Verification items for the finished model (mm, model axes). Give positions to 0.01 mm unless a question says otherwise; leave off trailing zeros. Write each loop counter-clockwise with the first axis right and the second up, starting at its lowest first coordinate (ties: lowest second). Pieces come first, ordered by that corner, then holes. Notation, with made-up numbers: (19.5, 65.5) -> (38.5, 65.5) arc R18 cw to (38.5, 90.5) -> close; hole circle Ø11 at (-14, -17). An arc over 180 degrees is marked (long way). Write item = value, one per line.
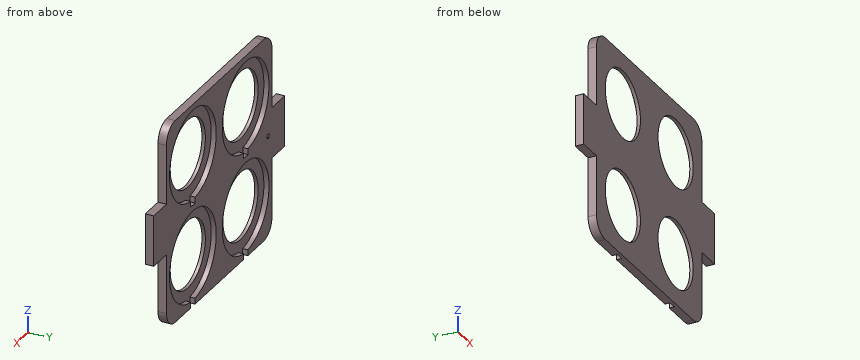
from build123d import *

# Parameters (mm, degrees)
SKETCH1_W           = 120
SKETCH1_H           = 120
BOSS_EXTRUDE1_DEPTH = 5
SKETCH2_R           = 20
CUT_EXTRUDE4_DEPTH  = 5
SKETCH3_R           = 26.6
SKETCH3_R_2         = 20
CUT_EXTRUDE5_DEPTH  = 3
SKETCH4_W           = 60
SKETCH4_H           = 5
BOSS_EXTRUDE2_DEPTH = 14.5
SKETCH5_W           = 60
SKETCH5_H           = 5
BOSS_EXTRUDE3_DEPTH = 14.5
FILLET3_R           = 10
FILLET4_R           = 10
FILLET5_R           = 10
FILLET6_R           = 10
SKETCH10_W          = 2.261137553
SKETCH10_H          = 2.574285836
CUT_EXTRUDE7_DEPTH  = 2
SKETCH12_W          = 5.377639696
SKETCH12_H          = 6.736845814
CUT_EXTRUDE10_DEPTH = 3
SKETCH14_W          = 4.90266265
SKETCH14_H          = 7.042630192
CUT_EXTRUDE11_DEPTH = 3
SKETCH15_W          = 14.5
SKETCH15_H          = 15
CUT_EXTRUDE12_DEPTH = 10


with BuildPart() as part:
    # Sketch1 → Boss-Extrude1 (new body)
    with BuildSketch(Plane(origin=(0, 0, 0), x_dir=(1, 0, 0), z_dir=(0, 1, 0))):
        Rectangle(SKETCH1_W, SKETCH1_H)
    extrude(amount=BOSS_EXTRUDE1_DEPTH)

    # Sketch2 → Cut-Extrude4 (cut)
    with BuildSketch(Plane(origin=(0, 5, 0), x_dir=(1, 0, 0), z_dir=(0, 1, 0))):
        with Locations(Location((30, 30, 0), (0, 0, 270))):
            Circle(SKETCH2_R)
        with Locations(Location((-30, -30, 0), (0, 0, 270))):
            Circle(SKETCH2_R)
        with Locations(Location((30, -30, 0), (0, 0, 270))):
            Circle(SKETCH2_R)
        with Locations(Location((-30, 30, 0), (0, 0, 270))):
            Circle(SKETCH2_R)
    extrude(amount=-CUT_EXTRUDE4_DEPTH, mode=Mode.SUBTRACT)

    # Sketch3 → Cut-Extrude5 (cut)
    # profile 1 of 4: a face of its own
    with BuildSketch(Plane(origin=(0, 5, 0), x_dir=(1, 0, 0), z_dir=(0, 1, 0))):
        with Locations(Location((30, 30, 0), (0, 0, 270))):
            Circle(SKETCH3_R)
        with Locations(Location((30, 30, 0), (0, 0, 270))):
            Circle(SKETCH3_R_2, mode=Mode.SUBTRACT)
    # profile 2 of 4: a face of its own
    with BuildSketch(Plane(origin=(0, 5, 0), x_dir=(1, 0, 0), z_dir=(0, 1, 0))):
        with Locations(Location((-30, -30, 0), (0, 0, 270))):
            Circle(SKETCH3_R)
        with Locations(Location((-30, -30, 0), (0, 0, 270))):
            Circle(SKETCH3_R_2, mode=Mode.SUBTRACT)
    # profile 3 of 4: a face of its own
    with BuildSketch(Plane(origin=(0, 5, 0), x_dir=(1, 0, 0), z_dir=(0, 1, 0))):
        with Locations(Location((30, -30, 0), (0, 0, 270))):
            Circle(SKETCH3_R)
        with Locations(Location((30, -30, 0), (0, 0, 270))):
            Circle(SKETCH3_R_2, mode=Mode.SUBTRACT)
    # profile 4 of 4: a face of its own
    with BuildSketch(Plane(origin=(0, 5, 0), x_dir=(1, 0, 0), z_dir=(0, 1, 0))):
        with Locations(Location((-30, 30, 0), (0, 0, 270))):
            Circle(SKETCH3_R)
    extrude(amount=-CUT_EXTRUDE5_DEPTH, mode=Mode.SUBTRACT)

    # Sketch4 → Boss-Extrude2 (add)
    with BuildSketch(Plane(origin=(60, 0, 0), x_dir=(0, 0, -1), z_dir=(1, 0, 0))):
        with Locations((0, 2.5)):
            Rectangle(SKETCH4_W, SKETCH4_H)
    extrude(amount=BOSS_EXTRUDE2_DEPTH)

    # Sketch5 → Boss-Extrude3 (add)
    with BuildSketch(Plane.ZY.offset(60)):
        with Locations((0, 2.5)):
            Rectangle(SKETCH5_W, SKETCH5_H)
    extrude(amount=BOSS_EXTRUDE3_DEPTH)

    # Fillet3
    fillet3_edges = [part.edges().sort_by_distance(p)[0] for p in [
        (-60, 2.5, 60),
    ]]
    fillet(fillet3_edges, radius=FILLET3_R)

    # Fillet4
    fillet4_edges = [part.edges().sort_by_distance(p)[0] for p in [
        (60, 2.5, 60),
    ]]
    fillet(fillet4_edges, radius=FILLET4_R)

    # Fillet5
    fillet5_edges = [part.edges().sort_by_distance(p)[0] for p in [
        (-60, 2.5, -60),
    ]]
    fillet(fillet5_edges, radius=FILLET5_R)

    # Fillet6
    fillet6_edges = [part.edges().sort_by_distance(p)[0] for p in [
        (60, 2.5, -60),
    ]]
    fillet(fillet6_edges, radius=FILLET6_R)

    # Sketch10 → Cut-Extrude7 (cut)
    with BuildSketch(Plane(origin=(0, 5, 0), x_dir=(1, 0, 0), z_dir=(0, 1, 0))):
        with Locations((-55.406362831, 0)):
            Rectangle(SKETCH10_W, SKETCH10_H)
    extrude(amount=-CUT_EXTRUDE7_DEPTH, mode=Mode.SUBTRACT)

    # Sketch12 → Cut-Extrude10 (cut)
    with BuildSketch(Plane(origin=(0, 5, 0), x_dir=(1, 0, 0), z_dir=(0, 1, 0))):
        with Locations((-30, -3.4)):
            Rectangle(SKETCH12_W, SKETCH12_H)
        with Locations((30, -3.4)):
            Rectangle(SKETCH12_W, SKETCH12_H)
    extrude(amount=-CUT_EXTRUDE10_DEPTH, mode=Mode.SUBTRACT)

    # Sketch14 → Cut-Extrude11 (cut)
    with BuildSketch(Plane(origin=(0, 5, 0), x_dir=(1, 0, 0), z_dir=(0, 1, 0))):
        with Locations((-30, 56.6)):
            Rectangle(SKETCH14_W, SKETCH14_H)
        with Locations((30, 56.6)):
            Rectangle(SKETCH14_W, SKETCH14_H)
    extrude(amount=-CUT_EXTRUDE11_DEPTH, mode=Mode.SUBTRACT)

    # Sketch15 → Cut-Extrude12 (cut)
    with BuildSketch(Plane(origin=(0, 5, 0), x_dir=(1, 0, 0), z_dir=(0, 1, 0))):
        with Locations((-67.25, 22.5)):
            Rectangle(SKETCH15_W, SKETCH15_H)
        with Locations((67.25, 22.5)):
            Rectangle(SKETCH15_W, SKETCH15_H)
        with Locations((67.25, -22.5)):
            Rectangle(SKETCH15_W, SKETCH15_H)
        with Locations((-67.25, -22.5)):
            Rectangle(SKETCH15_W, SKETCH15_H)
    extrude(amount=-CUT_EXTRUDE12_DEPTH, mode=Mode.SUBTRACT)


solid = part.part
Item 1: Material ranges on line 1 (X direction, y = 0.65, z = 30); line 2 (X direction, y = 3.15, z = -31.5); line 3 (Z direction, x = 21, y = 0.3), recorded low to high.
Response values:
line_1 = -60 to -50, -10 to 10, 50 to 60
line_2 = -60 to -56.56, -3.44 to 3.44, 56.56 to 60
line_3 = -60 to -47.86, -12.14 to 12.14, 47.86 to 60
Item 2: Sectioned sample at C-C on x = -13.5. Record the cut outline in (y, z).
Response values:
outline = (0, -60) -> (5, -60) -> (5, -50.86) -> (2, -50.86) -> (2, -41.3) -> (0, -41.3) -> close; (0, -18.7) -> (2, -18.7) -> (2, -9.14) -> (5, -9.14) -> (5, 9.14) -> (2, 9.14) -> (2, 18.7) -> (0, 18.7) -> close; (0, 41.3) -> (2, 41.3) -> (2, 50.86) -> (5, 50.86) -> (5, 60) -> (0, 60) -> close
Item 3: Sectioned sample at A-A on z = 30. Record the cut outline in (x, y), then the cut area to 3 significant figures.
Response values:
outline = (-60, 0) -> (-50, 0) -> (-50, 2) -> (-56.6, 2) -> (-56.6, 5) -> (-60, 5) -> close; (-10, 0) -> (10, 0) -> (10, 2) -> (3.4, 2) -> (3.4, 5) -> (-3.4, 5) -> (-3.4, 2) -> (-10, 2) -> close; (50, 0) -> (60, 0) -> (60, 5) -> (56.6, 5) -> (56.6, 2) -> (50, 2) -> close
area = 121 mm^2
Item 4: Sectioned sample at B-B on y = 1.1. Record the cut outline in (x, z), then the cut area to 3 significant figures.
Response values:
outline = (-74.5, -15) -> (-60, -15) -> (-60, -50) arc R10 ccw to (-50, -60) -> (50, -60) arc R10 ccw to (60, -50) -> (60, -15) -> (74.5, -15) -> (74.5, 15) -> (60, 15) -> (60, 50) arc R10 ccw to (50, 60) -> (-50, 60) arc R10 ccw to (-60, 50) -> (-60, 15) -> (-74.5, 15) -> close; hole circle Ø40 at (-30, -30); hole circle Ø40 at (-30, 30); hole circle Ø40 at (30, -30); hole circle Ø40 at (30, 30)
area = 10,200 mm^2
Item 5: Go/stop test with flat-tipped pins: P1, Ø10, axis at x = -30, z = 44.5, coming from the +Y side; P2, Ø2.5, axis at y = 3, z = -57.5, coming from the +X side; P3, Ø3, axis at y = 3.5, z = -31, coming from the -X side; P4, Ø2, axis at x = -55.5, y = 4.5, coming from the +Z side. Record where each tip stops, or that it passes through.
Response values:
P1 = through
P2 = 57.81
P3 = -60
P4 = 58.93
